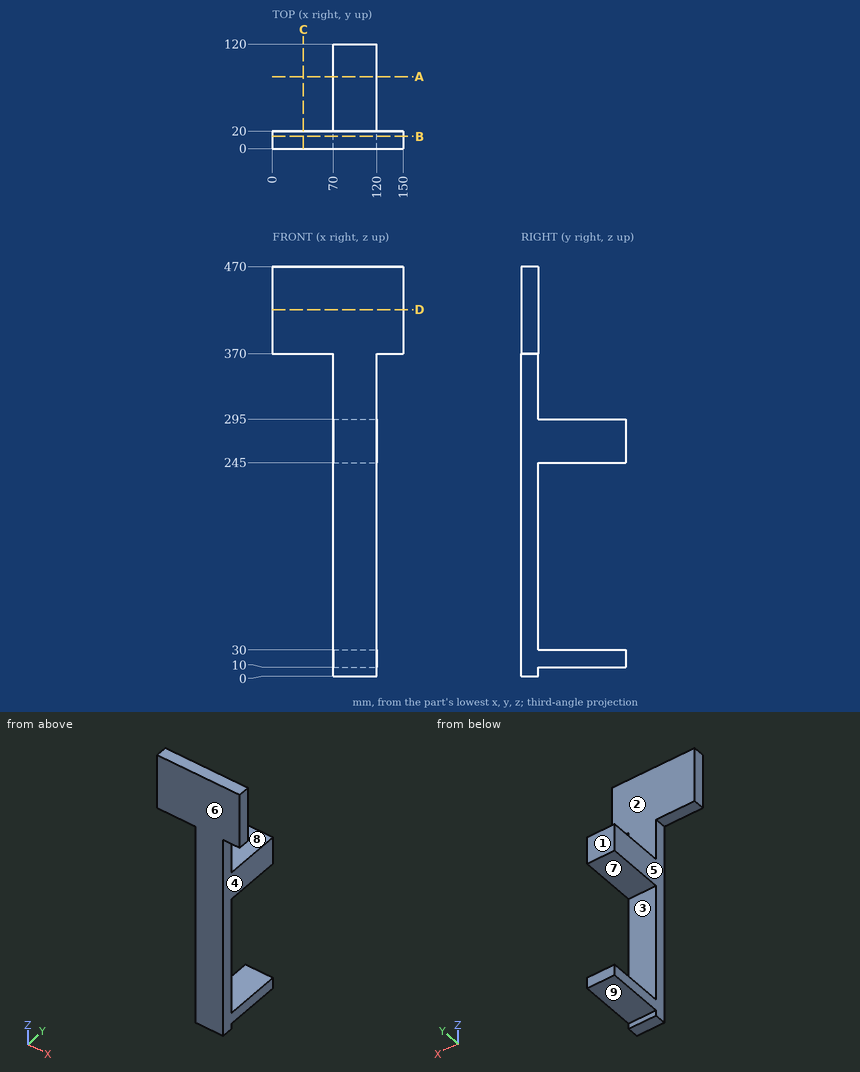
Drawing for the job (mm, zero at the part's lowest x, y, z). A direction names the side the tool comes from. Round coordinates to 2 decimals unless told otherwise and drop trailing zeros. Write each loop counter-clockwise with the first axis right and the second up, starting at its lowest first coordinate (ties: lowest second). Pieces come first, ordered by that corner, then holes. Notation, with made-up numbers: M 71,-18.75 L 88,-18.75 A35 cw 88,20.25 Z; hole C -35,26 d6. An arc over 180 degrees is marked long. One line per question, with ' | ' between items.
1. Cut at D-D on z = 420.5. Write the cut outline in (x, y).
Working result:
outline: M 0,0 L 150,0 L 150,20 L 0,20 Z
2. Cut at A-A on y = 82.5. Write the cut outline in (x, z).
Working result:
outline: M 70,10 L 120,10 L 120,30 L 70,30 Z; M 70,245 L 120,245 L 120,295 L 70,295 Z
3. Cut at C-C on x = 35.5. Write the cut outline in (y, z), and give its area (3 significant figures).
Working result:
outline: M 0,370 L 20,370 L 20,470 L 0,470 Z | area: 2,000 mm2
4. Mould opens along Z. For the marked faces 6, 7, 8 and 9 say: pulls with the +Z half, pulls with the -Z half, needs draft (parallel to the pull), parting line crosses it, or undercut.
Working result:
face 6: needs draft | face 7: undercut | face 8: pulls with the +Z half | face 9: pulls with the -Z half
5. Which spindle directions (+Z, -Z, +X, -X, +Y, -Y) get a long thin tool onto all of the face, cutting with end or side? Do the marked faces 1, 2, 3, 4 and 5. Say none if no direction does.
Working result:
face 1: +Z, -Z, +X, -X, +Y | face 2: +Z, +X, -X, +Y | face 3: +X, -X, +Y | face 4: -Z, +X, +Y, -Y | face 5: -Z, -X, +Y, -Y
6. Cut at B-B on y = 14. Write the cut outline in (x, z), and give its area (3 significant figures).
Working result:
outline: M 0,370 L 70,370 L 70,0 L 120,0 L 120,370 L 150,370 L 150,470 L 0,470 Z | area: 33,500 mm2
7. Pin check, flat tips, straight feed: pin 1 Ø10 at (x, y) = (141, 9) entering from -Z; pin 2 Ø2 at (x, z) = (120, 228) entering from +Y; pin 3 Ø1 at (y, z) = (44, 268) entering from -X. Stop position of each tip, or through.
Working result:
pin 1: z = 370 | pin 2: y = 20 | pin 3: x = 70
8. Probe L1, parallel to Z at x = 100, y = 30; L2, parallel to Z at x = 122.5, y = 7; L3, parallel to X at y = 68.5, z = 284.5. List the from-to ranges inside material, lowest first. Write a range as from..to.
Working result:
L1: 10..30, 245..295 | L2: 370..470 | L3: 70..120
